For this review, take the finished solid that the model builds, in its own axes (mm). Face numbers are marked on the shaded views. A direction names the side the tool comes from. Coordinates: 2 decimals unless noted, no trailing zeros. Write each loop counter-clockwise with the first axis right and the second up, starting at its lowest first coordinate (ties: lowest second). Pieces come first, ordered by that corner, then holes. Notation, with made-up numbers: M 82.5,2.5 L 136.5,2.5 A16 cw 136.5,15.5 Z; hole C 1,44.5 d11. An arc over 180 degrees is marked long. One line per question, with ' | ' between items.
Solid Edge part; units mm, degrees
sketch "Sketch1" plane through (0, 0, 0) normal (1, 0, 0) x (0, 1, 0)
  line L0 (-50, 0) -> (-20, 62)
  line L1 (-20, 62) -> (20, 62)
  line L2 (50, 0) -> (20, 62)
  line L3 (50, 0) -> (79.8022, 0)
  line L4 (79.8022, 0) -> (79.8022, 5)
  line L5 (79.8022, 5) -> (57.8022, 5)
  line L6 (25, 67) -> (57.8022, 5)
  line L7 (-25, 67) -> (25, 67)
  line L8 (-55, 5) -> (-25, 67)
  line L9 (-77, 5) -> (-55, 5)
  line L10 (-77, 0) -> (-77, 5)
  line L11 (-77, 0) -> (-50, 0)
  dimension "D1" = 20
  dimension "D2" = 79.8022
  dimension "D3" = 79.8022
  dimension "D4" = 77
  dimension "D5" = 25
  dimension "D6" = 77
extrude "Protrusion1" add sketch "Sketch1" along normal blind 50
sketch "Sketch2" plane through (25, 0, 67) normal (0, 0, 1) x (1, 0, 0)
  line L0 (-25, 20) -> (25, 20)
  line L1 (25, 20) -> (25, 15)
  line L2 (25, 15) -> (-25, 15)
  line L3 (-25, 15) -> (-25, 20)
  line L4 (-25, -20) -> (25, -20)
  line L5 (25, -20) -> (25, -15)
  line L6 (25, -15) -> (-25, -15)
  line L7 (-25, -15) -> (-25, -20)
  dimension "D1" = 25
extrude "ExtrudedProtrusion_2" add sketch "Sketch2" along normal blind 2.5
sketch "Sketch3" plane through (25, -66, 5) normal (0, 0, 1) x (1, 0, 0)
  circle A0 centre (-12.5, -2) radius 4
  circle A1 centre (12.5, -2) radius 4
  dimension "D1" = 12.5
extrude "Cutout1" cut sketch "Sketch3" against normal up to next
mirror "Mirror1" about plane through (0, 0, 0) normal (0, -1, 0) of "Cutout1"
sketch "Sketch4" plane through (25, 0, 67) normal (0, 0, 1) x (0, 1, 0)
  circle A0 centre (0, 15) radius 2.5
  circle A1 centre (0, -17.5) radius 2.5
extrude "Cutout2" cut sketch "Sketch4" against normal up to next
sketch "Sketch5" plane through (0, 0, 0) normal (0, 1, 0) x (-1, 0, 0)
  line L0 (0, 0) -> (-66.0658, 1.6838)
  line L1 (-66.0658, 1.6838) -> (-66.0658, 0)
  line L2 (-66.0658, 0) -> (0, 0)
extrude "ExtrudedCutout_3" cut sketch "Sketch5" along normal mid plane 208
fillet "Round_1" radius 5 7 edges at (25, 25, 67) (25, 49.6917, 0.6372) (25, 57.8022, 5) (25, -25, 67) (25, -20, 62) (25, -49.6917, 0.6372) (25, -55, 5)
sketch "Sketch6" plane through (25, 41.4011, 36) normal (0, 0.8839, 0.4677) x (-1, 0, 0)
  circle A0 centre (0, 17.06) radius 10
  circle A1 centre (0, -12.94) radius 10
extrude "Cutout3" cut sketch "Sketch6" against normal up to next
mirror "Mirror2" about plane through (0, 0, 0) normal (0, -1, 0) of "Cutout3"
properties material "Stainless steel"
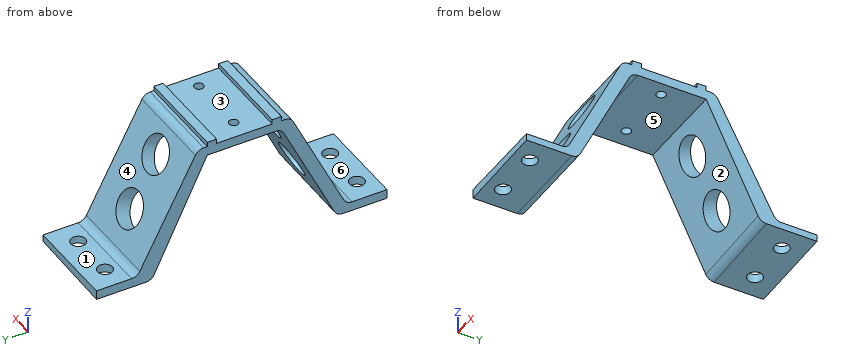
1) Insertion check: pin 1 Ø2 at (x, y) = (27, 43.5) entering from +Z; pin 2 Ø1 at (x, y) = (9.5, -38) entering from +Z; pin 3 Ø2 at (x, z) = (36.5, 69) entering from +Y; pin 4 Ø10 at (y, z) = (-26.5, 42) entering from -X. Each pin has a flat end and moves straight along its axis. Give the tip position at first contact, or say it passes through.
Responses:
pin 1: z = 33.92 | pin 2: z = 41.17 | pin 3: y = 20 | pin 4: x = 0
2) The part is to be moulded in two halves that separate along Y. For the marked faces 4, 5 and 6, say which applies: +Y half, -Y half, draft (parallel to the pull), parting line (faces both ways), or undercut.
Responses:
face 4: +Y half | face 5: undercut | face 6: draft
3) We need section C-C on x = 27.5. State how many separate pieces and enclosed holes the cut face has, then the cut area to 3 significant figures.
Responses:
separate pieces: 5 | enclosed holes: 0 | area: 910 mm^2
4) We need section D-D on y = -13. State the section outline as (x, z) points.
Responses:
outline: M 0,62 L 50,62 L 50,67 L 0,67 Z
5) Machinability: for the marked faces 1, 2 and 3, which of the approach directions +Z, -Z, +X, -X, +Y, -Y give a long, thin tool a straight path to every point of the face, cutting with its end or side? Answer none if there is none.
Responses:
face 1: +Z, +X, -X, +Y | face 2: -Z, +X, -X | face 3: +Z, +X, -X
6) To check wall thickness, follow line 1 along X through (y, z) = (-68, 3); line 2 along Y through (x, z) = (37.5, 4.1); line 3 along X through (y, z) = (0, 65). State the ranges of each line that lie inside material, in increasing order. Write a range as [from, to].
Responses:
line 1: [0, 8.5], [16.5, 33.5], [41.5, 50] | line 2: [-77, -72], [-64, -48.02], [48.02, 64], [72, 79.8] | line 3: [0, 7.5], [12.5, 40], [45, 50]
7) We need section A-A on y = 68. State the section outline as (x, z) points.
Responses:
outline: M 0,0 L 8.5,0.22 L 8.5,5 L 0,5 Z; M 16.5,0.42 L 33.5,0.85 L 33.5,5 L 16.5,5 Z; M 41.5,1.06 L 50,1.27 L 50,5 L 41.5,5 Z
8) We need section B-B on z = 9.5. State the section outline as (x, y) points.
Responses:
outline: M 0,-52.82 L 50,-52.82 L 50,-45.4 L 0,-45.4 Z; M 0,45.4 L 50,45.4 L 50,55.42 L 0,55.42 Z
